from build123d import *

# Parameters (mm, degrees)
SKETCH_1_R          = 4.25
EXTRUDE_1_DEPTH     = 32.35
SKETCH_2_R          = 3
EXTRUDE_2_DEPTH     = 1
SKETCH_3_R          = 2.5
EXTRUDE_3_DEPTH     = 4
EXTRUDE_START       = 4
SKETCH_4_R          = 3
EXTRUDE_4_DEPTH     = 4
SKETCH_5_R          = 2.5
EXTRUDE_5_DEPTH     = 4
CHAMFER_1_SIZE      = 0.5
CHAMFER_2_SIZE      = 0.5
SKETCH_6_W          = 6
SKETCH_6_H          = 3
CUT_EXTRUDE_6_DEPTH = 7.5
CHAMFER1_SIZE       = 1


with BuildPart() as part:
    # 草图1 → 拉伸1 (new, symmetric)
    with BuildSketch(Plane.XY):
        with Locations(Location((0, 0, 0), (0, 0, 180))):
            Circle(SKETCH_1_R)
    extrude(amount=EXTRUDE_1_DEPTH, both=True)

    # 草图2 → 拉伸2 (add)
    with BuildSketch(Plane.XY.offset(32.35)):
        Circle(SKETCH_2_R)
    extrude(amount=EXTRUDE_2_DEPTH)

    # 草图3 → 拉伸3 (add)
    with BuildSketch(Plane.XY.offset(33.35)):
        Circle(SKETCH_3_R)
    extrude(amount=EXTRUDE_3_DEPTH)

    # 草图4 → 拉伸4 (add)
    with BuildSketch(Plane(origin=(0, 0, -32.35), x_dir=(-1, 0, 0), z_dir=(0, 0, -1)).offset(EXTRUDE_START)):
        with Locations(Location((0, 0, 0), (0, 0, 180))):
            Circle(SKETCH_4_R)
    extrude(amount=-EXTRUDE_4_DEPTH)

    # 草图5 → 拉伸5 (add)
    with BuildSketch(Plane(origin=(0, 0, -36.35), x_dir=(-1, 0, 0), z_dir=(0, 0, -1)).offset(EXTRUDE_START)):
        with Locations(Location((0, 0, 0), (0, 0, 180))):
            Circle(SKETCH_5_R)
    extrude(amount=-EXTRUDE_5_DEPTH)

    # 倒角1
    chamfer_1_edges = [part.edges().sort_by_distance(p)[0] for p in [
        (-2.5, 0, 37.35),
        (-2.5, 0, -40.35),
    ]]
    chamfer(chamfer_1_edges, length=CHAMFER_1_SIZE)

    # 倒角2
    chamfer_2_edges = [part.edges().sort_by_distance(p)[0] for p in [
        (-3, 0, -36.35),
    ]]
    chamfer(chamfer_2_edges, length=CHAMFER_2_SIZE - 0.0001)  # a hair under: the kernel refuses the full size

    # 草图6 → 拉伸6 (cut)
    with BuildSketch(Plane(origin=(0, 0, -40.35), x_dir=(-1, 0, 0), z_dir=(0, 0, -1))):
        with Locations((0, 3.5)):
            Rectangle(SKETCH_6_W, SKETCH_6_H)
    extrude(amount=-CUT_EXTRUDE_6_DEPTH, mode=Mode.SUBTRACT)

    # Chamfer1
    chamfer1_edges = [part.edges().sort_by_distance(p)[0] for p in [
        (4.25, 0, -32.35),
        (4.25, 0, 32.35),
    ]]
    chamfer(chamfer1_edges, length=CHAMFER1_SIZE)


solid = part.part
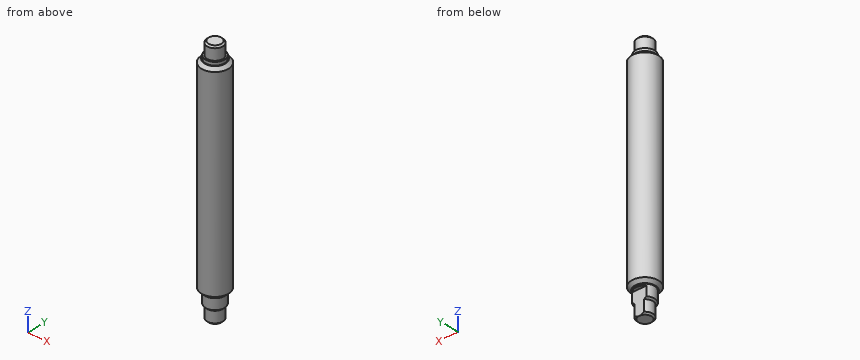
Can you work these out from the model? Positions are in its coordinate system, mm. Give positions to 0.01 mm unless a question says otherwise; leave off trailing zeros. Loops run counter-clockwise (first coordinate to the right, second up) from the corner with the lowest first, then second, coordinate; pieces in that order, holes last. Notation, with made-up numbers: (28.25, 76) -> (84.25, 76) arc R5 ccw to (84.25, 82) -> close; hole circle Ø4 at (-12, -13.75). An arc over 180 degrees is marked (long way). Write item = value, one per line.
1) Will these pins go through, and if not, where does the flat tip stop? pin 1 (1.3 mm diameter, centred on x = -1, z = -38, fed in from +Y); pin 2 (0.5 mm diameter, centred on x = 1, y = 2.5, fed in from -Z); pin 3 (4 mm diameter, centred on y = 3.5, z = 0.5, fed in from +X).
Check result:
pin_1 = 2
pin_2 = -32.85
pin_3 = 3.98
2) I need wall thicknesses on L1, parallel to Y at x = 0, z = -35.5; L2, parallel to Z at x = 1.5, y = 2.5; L3, parallel to X at y = -2.75, z = -8.5. Which ranges of each line are inside material? Lowest first, please. Write a range as from..to.
Check result:
L1 = -3..2
L2 = -32.85..33.35
L3 = -3.24..3.24
3) Suppose I cut it at A-A on z = 1. Write out the boundary of the cut face in (x, y).
Check result:
outline = circle Ø8.5 at (0, 0)
